Here's how the part is built. I have some questions about the finished solid (model axes, mm). A direction names the side the tool comes from. Coordinates: 2 decimals unless noted, no trailing zeros. Order: outer loops, then holes, each group sorted by start corner. A loop starts at its lowest first (then second) coordinate and runs counter-clockwise, first axis right, second up. Notation, with made-up numbers: (-9, 13.5) -> (-5, 13.5) arc R25 cw to (-5, 45.5) -> close; hole circle Ø11 at (4, 42.25). An arc over 180 degrees is marked (long way). One line per item, written item: value. Start each with the question number.
Autodesk Inventor part; units mm, degrees
ref_plane "YZ Plane" through (0, 0, 0) normal (1, 0, 0) x (0, 1, 0)
ref_plane "XZ Plane" through (0, 0, 0) normal (0, 1, 0) x (-1, 0, 0)
ref_plane "XY Plane" through (0, 0, 0) normal (0, 0, 1) x (1, 0, 0)
sketch "Sketch1" plane through (0, 0, 0) normal (0, 0, 1) x (1, 0, 0)
  line L0 (-170, 50) -> (170, 50)
  line L1 (170, 50) -> (170, -50)
  line L2 (170, -50) -> (-170, -50)
  line L3 (-170, -50) -> (-170, 50)
  point P0 (0, 0)
  dimension "d0" = 340
  dimension "d1" = 170
  dimension "d2" = 100
  dimension "d3" = 50
extrude "baseExtrusion" add sketch "Sketch1" along normal blind 10
sketch "Sketch2" plane through (0, 0, 10) normal (0, 0, 1) x (1, 0, 0)
  line L0 (170, 50) -> (-170, 50)
  line L1 (-170, 50) -> (-170, -50)
  point P0 (0, 0)
  point P1 (-155, 35)
  dimension "d6" = 15
  dimension "d7" = 15
hole "xyStiltpt1m6MountingHoles" at (-155, 35, 10) direction (0, 0, -1) diameter 4.917 end through all
mirror "Mirror2" about plane through (0, 0, 0) normal (1, 0, 0) of "xyStiltpt1m6MountingHoles"
mirror "Mirror3" about plane through (0, 0, 0) normal (0, 1, 0) of "xyStiltpt1m6MountingHoles", "Mirror2"
sketch "Sketch4" plane through (0, 0, 0) normal (0, 0, -1) x (-1, 0, 0)
  line L0 (170, -50) -> (170, 50)
  line L1 (170, 50) -> (-170, 50)
  line L2 (-170, 50) -> (-170, -50)
  line L3 (-170, -50) -> (170, -50)
  point P0 (0, 0)
  point P1 (155, 0)
  point P2 (0, 0)
  point P3 (0, 35)
  point P4 (0, -35)
  point P5 (-155, 0)
  dimension "d24" = 15
  dimension "d25" = 15
  dimension "d26" = 15
  dimension "d27" = 15
hole "Hole3" at (-155, 0, 0) at (0, 0, 0) at (0, 35, 0) at (0, -35, 0) at (155, 0, 0) direction (0, 0, 1) diameter 6.6 end through all counterbore diameter 18 counterbore depth 4.8
properties part number "xyStageStilt_pt2"
Q1. Imagine slicing it at B-B (x = 0). Write out the boundary of the cut face in (y, z), plus the area to 3 significant figures.
Q2. Imagine slicing it at C-C (z = 1.5). Count the separate pieces of the cut face and the enclosed holes in it, plus the area to 3 significant figures.
Q3. For faces 1 (the face through (4, 0, 4.8)), 2 (the face through (170, 1, 5)), which set-ups out of +Z, -Z, +X, -X, +Y, -Y let a thin tool reach every point of the face, with its end or its side?
Q4. If we mould it in two halves opening along Y, with no side actions, what happens to faces 3 (the face through (-2.23, -2.43, 7.44)), 4 (the face through (2, -50, 5)), 5 (the face through (-163.923, -1.172, 2.434)), 6 (the face through (-2, 50, 5))? For each: +Y half, -Y half, draft (parallel to the pull), parting line (faces both ways), or undercut.
Q5. For P1, Ø5.5, axis at x = 2, y = -34, coming from the -Z side, with a flat end and sliding along its axis, tell me the tip position at first contact or that it passes through.
Q6. Imagine slicing it at A-A (y = 0). Write out the boundary of the cut face in (x, z).
Q7. I need wall thicknesses on line 1 (X direction, y = 0, z = 6); line 2 (Y direction, x = -155, z = 2.6); line 3 (Y direction, x = 0, z = 7.4). Which ranges of each line are inside material? Lowest first, please.
Completed:
1. outline: (-50, 0) -> (-44, 0) -> (-44, 4.8) -> (-38.3, 4.8) -> (-38.3, 10) -> (-50, 10) -> close; (-31.7, 4.8) -> (-26, 4.8) -> (-26, 0) -> (-9, 0) -> (-9, 4.8) -> (-3.3, 4.8) -> (-3.3, 10) -> (-31.7, 10) -> close; (3.3, 4.8) -> (9, 4.8) -> (9, 0) -> (26, 0) -> (26, 4.8) -> (31.7, 4.8) -> (31.7, 10) -> (3.3, 10) -> close; (38.3, 4.8) -> (44, 4.8) -> (44, 0) -> (50, 0) -> (50, 10) -> (38.3, 10) -> close
1. area: 638 mm2
2. separate pieces: 1
2. enclosed holes: 9
2. area: 32,700 mm2
3. face 1: -Z
3. face 2: +Z, -Z, +X, +Y, -Y
4. face 3: undercut
4. face 4: -Y half
4. face 5: undercut
4. face 6: +Y half
5. P1: stops at z = 4.8
6. outline: (-170, 0) -> (-164, 0) -> (-164, 4.8) -> (-158.3, 4.8) -> (-158.3, 10) -> (-170, 10) -> close; (-151.7, 4.8) -> (-146, 4.8) -> (-146, 0) -> (-9, 0) -> (-9, 4.8) -> (-3.3, 4.8) -> (-3.3, 10) -> (-151.7, 10) -> close; (3.3, 4.8) -> (9, 4.8) -> (9, 0) -> (146, 0) -> (146, 4.8) -> (151.7, 4.8) -> (151.7, 10) -> (3.3, 10) -> close; (158.3, 4.8) -> (164, 4.8) -> (164, 0) -> (170, 0) -> (170, 10) -> (158.3, 10) -> close
7. line 1: x = -170 to -158.3, -151.7 to -3.3, 3.3 to 151.7, 158.3 to 170
7. line 2: y = -50 to -37.46, -32.54 to -9, 9 to 32.54, 37.46 to 50
7. line 3: y = -50 to -38.3, -31.7 to -3.3, 3.3 to 31.7, 38.3 to 50
